```python
from build123d import *

# Parameters (mm, degrees)
F0_W     = 165.1
F0_H     = 165.1
F0_W_2   = 1.5875
F1_DEPTH = 1.1811
F2_R     = 4.3688
F3_DEPTH = 1.1811
F4_R     = 5.08
F5_R     = 2.54
F6_DEPTH = 1.1811


with BuildPart() as f1:
    # F0 (on Top) → F1 (new body)
    with BuildSketch(Plane.XY):
        with Locations((0, 82.55)):
            Rectangle(F0_W, F0_H)
        with Locations((-83.34375, 82.55)):
            Rectangle(F0_W_2, F0_H)
        with Locations((83.34375, 82.55)):
            Rectangle(F0_W_2, F0_H)
        with BuildLine():
            Line((-82.55, 273.05), (-82.55, 165.1))
            Line((-82.55, 165.1), (82.55, 165.1))
            Line((82.55, 165.1), (82.55, 273.05))
            Line((82.55, 273.05), (34.925, 273.05))
            Line((34.925, 273.05), (34.925, 239.8014))
            ThreePointArc((34.925, 239.8014), (0, 204.8764), (-34.925, 239.8014))
            Line((-34.925, 239.8014), (-34.925, 273.05))
            Line((-34.925, 273.05), (-82.55, 273.05))
        make_face()
        Polygon((-261.9375, 0), (-84.1375, 0), (-84.1375, 165.1), (-190.5, 165.1), (-190.5, 63.5), (-261.9375, 63.5), align=None)
        Polygon((84.1375, 165.1), (84.1375, 0), (261.9375, 0), (261.9375, 63.5), (190.5, 63.5), (190.5, 165.1), align=None)
    extrude(amount=F1_DEPTH)

    # F2 (on face) → F3 (cut, through all)
    with BuildSketch(Plane.XY.offset(1.1811)):
        with Locations((-57.15, 19.05)):
            Circle(F2_R)
        with Locations((57.15, 19.05)):
            Circle(F2_R)
        with BuildLine():
            ThreePointArc((-28.0416, 104.8004), (-33.3502, 110.109), (-38.6588, 104.8004))
            Line((-38.6588, 104.8004), (-38.6588, 74.6252))
            ThreePointArc((-38.6588, 74.6252), (-33.3502, 69.3166), (-28.0416, 74.6252))
            Line((-28.0416, 74.6252), (-28.0416, 104.8004))
        make_face()
        with BuildLine():
            ThreePointArc((-5.3086, 74.6252), (0, 69.3166), (5.3086, 74.6252))
            Line((5.3086, 74.6252), (5.3086, 104.8004))
            ThreePointArc((5.3086, 104.8004), (0, 110.109), (-5.3086, 104.8004))
            Line((-5.3086, 104.8004), (-5.3086, 74.6252))
        make_face()
        with BuildLine():
            ThreePointArc((38.6588, 104.8004), (33.3502, 110.109), (28.0416, 104.8004))
            Line((28.0416, 104.8004), (28.0416, 74.6252))
            ThreePointArc((28.0416, 74.6252), (33.3502, 69.3166), (38.6588, 74.6252))
            Line((38.6588, 74.6252), (38.6588, 104.8004))
        make_face()
    extrude(amount=-F3_DEPTH, mode=Mode.SUBTRACT)

    # F4
    f4_edges = [f1.edges().sort_by_distance(p)[0] for p in [
        (-82.55, 273.05, 0.59055),
        (-34.925, 273.05, 0.59055),
        (34.925, 273.05, 0.59055),
        (82.55, 273.05, 0.59055),
        (190.5, 165.1, 0.59055),
        (261.9375, 63.5, 0.59055),
        (190.5, 63.5, 0.59055),
        (261.9375, 0, 0.59055),
        (-261.9375, 0, 0.59055),
        (-261.9375, 63.5, 0.59055),
        (-190.5, 63.5, 0.59055),
        (-190.5, 165.1, 0.59055),
    ]]
    fillet(f4_edges, radius=F4_R)

    # F5 (on face) → F6 (cut, through all)
    with BuildSketch(Plane.XY.offset(1.1811)):
        with BuildLine():
            ThreePointArc((-80.9625, 146.05), (-82.55, 147.6375), (-84.1375, 146.05))
            Line((-84.1375, 146.05), (-84.1375, 127))
            ThreePointArc((-84.1375, 127), (-82.55, 125.4125), (-80.9625, 127))
            Line((-80.9625, 127), (-80.9625, 146.05))
        make_face()
        with BuildLine():
            ThreePointArc((-80.9625, 107.95), (-82.55, 109.5375), (-84.1375, 107.95))
            Line((-84.1375, 107.95), (-84.1375, 88.9))
            ThreePointArc((-84.1375, 88.9), (-82.55, 87.3125), (-80.9625, 88.9))
            Line((-80.9625, 88.9), (-80.9625, 107.95))
        make_face()
        with BuildLine():
            ThreePointArc((-80.9625, 69.85), (-82.55, 71.4375), (-84.1375, 69.85))
            Line((-84.1375, 69.85), (-84.1375, 50.8))
            ThreePointArc((-84.1375, 50.8), (-82.55, 49.2125), (-80.9625, 50.8))
            Line((-80.9625, 50.8), (-80.9625, 69.85))
        make_face()
        with BuildLine():
            ThreePointArc((-80.9625, 31.75), (-82.55, 33.3375), (-84.1375, 31.75))
            Line((-84.1375, 31.75), (-84.1375, 12.7))
            ThreePointArc((-84.1375, 12.7), (-82.55, 11.1125), (-80.9625, 12.7))
            Line((-80.9625, 12.7), (-80.9625, 31.75))
        make_face()
        with BuildLine():
            Line((84.1375, 127), (84.1375, 146.05))
            ThreePointArc((84.1375, 146.05), (82.55, 147.6375), (80.9625, 146.05))
            Line((80.9625, 146.05), (80.9625, 127))
            ThreePointArc((80.9625, 127), (82.55, 125.4125), (84.1375, 127))
        make_face()
        with BuildLine():
            Line((80.9625, 107.95), (80.9625, 88.9))
            ThreePointArc((80.9625, 88.9), (82.55, 87.3125), (84.1375, 88.9))
            Line((84.1375, 88.9), (84.1375, 107.95))
            ThreePointArc((84.1375, 107.95), (82.55, 109.5375), (80.9625, 107.95))
        make_face()
        with BuildLine():
            Line((84.1375, 50.8), (84.1375, 69.85))
            ThreePointArc((84.1375, 69.85), (82.55, 71.4375), (80.9625, 69.85))
            Line((80.9625, 69.85), (80.9625, 50.8))
            ThreePointArc((80.9625, 50.8), (82.55, 49.2125), (84.1375, 50.8))
        make_face()
        with BuildLine():
            Line((80.9625, 31.75), (80.9625, 12.7))
            ThreePointArc((80.9625, 12.7), (82.55, 11.1125), (84.1375, 12.7))
            Line((84.1375, 12.7), (84.1375, 31.75))
            ThreePointArc((84.1375, 31.75), (82.55, 33.3375), (80.9625, 31.75))
        make_face()
        with BuildLine():
            ThreePointArc((-66.675, 166.6875), (-68.2625, 165.1), (-66.675, 163.5125))
            Line((-66.675, 163.5125), (-50.165, 163.5125))
            ThreePointArc((-50.165, 163.5125), (-48.5775, 165.1), (-50.165, 166.6875))
            Line((-50.165, 166.6875), (-66.675, 166.6875))
        make_face()
        with BuildLine():
            ThreePointArc((-37.465, 166.6875), (-39.0525, 165.1), (-37.465, 163.5125))
            Line((-37.465, 163.5125), (-20.955, 163.5125))
            ThreePointArc((-20.955, 163.5125), (-19.3675, 165.1), (-20.955, 166.6875))
            Line((-20.955, 166.6875), (-37.465, 166.6875))
        make_face()
        with BuildLine():
            ThreePointArc((-8.255, 166.6875), (-9.8425, 165.1), (-8.255, 163.5125))
            Line((-8.255, 163.5125), (8.255, 163.5125))
            ThreePointArc((8.255, 163.5125), (9.8425, 165.1), (8.255, 166.6875))
            Line((8.255, 166.6875), (-8.255, 166.6875))
        make_face()
        with BuildLine():
            ThreePointArc((20.955, 166.6875), (19.3675, 165.1), (20.955, 163.5125))
            Line((20.955, 163.5125), (37.465, 163.5125))
            ThreePointArc((37.465, 163.5125), (39.0525, 165.1), (37.465, 166.6875))
            Line((37.465, 166.6875), (20.955, 166.6875))
        make_face()
        with BuildLine():
            ThreePointArc((50.165, 166.6875), (48.5775, 165.1), (50.165, 163.5125))
            Line((50.165, 163.5125), (66.675, 163.5125))
            ThreePointArc((66.675, 163.5125), (68.2625, 165.1), (66.675, 166.6875))
            Line((66.675, 166.6875), (50.165, 166.6875))
        make_face()
        with Locations((-82.55, 165.1)):
            Circle(F5_R)
        with Locations((82.55, 165.1)):
            Circle(F5_R)
    extrude(amount=-F6_DEPTH, mode=Mode.SUBTRACT)


solid = f1.part
```
Verification items for the finished model (mm, model axes). Coordinates: 2 decimals unless noted, no trailing zeros. Order: outer loops, then holes, each group sorted by start corner. A loop starts at its lowest first (then second) coordinate and runs counter-clockwise, first axis right, second up. Notation, with made-up numbers: (18.5, 75.25) -> (26.5, 75.25) arc R19 ccw to (26.5, 103.25) -> close; hole circle Ø2 at (34, 81.25). An arc over 180 degrees is marked (long way). Answer as CSV lines item,"result". Start each with the question number.
1) Release check for a two-part mould opening along X. For faces 1 (the face through (0.768, 204.885, 0.582)), 2 (the face through (-4, 138, 0)) record: released by +X, released by -X, zero draft, split by the parting line, or undercut.
2) Cross-section at A-A, the plane x = 0. Record the boundary of the cut face in (y, z).
3) Cross-section at D-D, the plane x = 175.5. Record the boundary of the cut face in (y, z), then the cut area to 3 significant figures.
4) Gauge pin test, flat ends, axial feed: pin 1 Ø4.5 at (x, y) = (82.55, 165.1) entering from +Z; pin 2 Ø0.6 at (y, z) = (85, 0.5) entering from -X; pin 3 Ø0.6 at (y, z) = (94, 0.5) entering from +X. Record the tip position at first contact, or that the pin passes through.
5) Cross-section at B-B, the plane z = 0.4. Give the number of separate pieces and of enclosed holes in the cut face, then the cut area to 3 significant figures.
6) Material ranges on L1, parallel to Y at x = -57.15, z = 0.8; L2, parallel to X at y = 139.5, z = 0.45; L3, parallel to Y at x = 38, z = 0.6, recorded low to high. Write a range as [from, to].
7) Cross-section at C-C, the plane x = -226. Record the boundary of the cut face in (y, z), then the cut area to 3 significant figures.
Conclusion:
1,face 1,"undercut"
1,face 2,"zero draft"
2,outline,"(0, 0) -> (69.32, 0) -> (69.32, 1.18) -> (0, 1.18) -> close; (110.11, 0) -> (163.51, 0) -> (163.51, 1.18) -> (110.11, 1.18) -> close; (166.69, 0) -> (204.88, 0) -> (204.88, 1.18) -> (166.69, 1.18) -> close"
3,outline,"(0, 0) -> (165.1, 0) -> (165.1, 1.18) -> (0, 1.18) -> close"
3,area,"195 mm²"
4,pin 1,"passes through"
4,pin 2,"stops at x = -190.5"
4,pin 3,"stops at x = 190.5"
5,separate pieces,"1"
5,enclosed holes,"18"
5,area,"83,300 mm²"
6,L1,"y = [0, 14.68], [23.42, 163.51], [166.69, 273.05]"
6,L2,"x = [-190.5, -84.14], [-80.96, 80.96], [84.14, 190.5]"
6,L3,"y = [0, 72.06], [107.36, 163.61], [166.59, 272.64]"
7,outline,"(0, 0) -> (63.5, 0) -> (63.5, 1.18) -> (0, 1.18) -> close"
7,area,"75.0 mm²"
